Read the model definition and answer for the solid it produces. Units are mm, in the model's axes. A direction names the side the tool comes from. Round coordinates to 2 decimals unless told otherwise and drop trailing zeros. Order: outer loops, then holes, each group sorted by start corner. A loop starts at its lowest first (then second) coordinate and runs counter-clockwise, first axis right, second up. Notation, with made-up numbers: (84.5, 6) - (93.5, 6) arc R26 cw to (93.5, 26) - close; hole circle Ø5 at (-31, 52). An arc over 180 degrees is marked (long way). One line per question, with ' | ' between items. Start each with the question number.
1) The part is cut by section A-A, the plane y = -242.5. Give the vertices of the cut face in (x, z), plus the area to 3 significant figures.
2) Flat-ended cylindrical pins translate along their axes: pin 1 (5 mm diameter, centred on x = 10.5, z = 71.5, fed in from +Y); pin 2 (3 mm diameter, centred on x = -21, z = 16.5, fed in from +Y); pin 3 (21 mm diameter, centred on x = -3.5, z = 47, fed in from +Y); pin 4 (6 mm diameter, centred on x = 0, y = -400, fed in from +Z). Find the tip coordinate at first contact, or state that the pin passes through.
3) Straight lines are drawn through the part: line 1 (X direction, y = -400, z = 82.25); line 2 (Y direction, x = -5.5, z = 64); line 3 (Z direction, x = 3.5, y = -175). For each, find the intervals that lie inside material, in ascending order. Write a range as from..to.
4) The mould has two halves that part along Y. Classify faces 1 (the flat face through (0, -186, 15)), 2 (the cylindrical face through (0, -420, 82)), 3 (the flat face through (0, -192, 0)): pulls with the +Y half, pulls with the -Y half, needs draft (parallel to the pull), parting line crosses it, or undercut.
5) For faces 4 (the flat face through (0, -323, 75)), 5 (the flat face through (0, -192, 90)), 6 (the flat face through (0, -390, 75)), determine the directions among +Z, -Z, +X, -X, +Y, -Y from which every point of the face is accessible in a straight line to the end or side of a thin tool.
6) The part is cut by section D-D, the plane z = 5.5. Give the vertices of the cut face in (x, y), plus the area to 3 significant figures.
7) The part is cut by section B-B, the plane z = 26.5. Give the vertices of the cut face in (x, y).
8) The part is cut by section C-C, the plane x = 0. Count the separate pieces of the cut face and the enclosed holes in it, plus the area to 3 significant figures.
from build123d import *

# Parameters (mm, degrees)
SKETCH_1_R               = 5
EXTRUDE_1_DEPTH          = 90
CUT_EXTRUDE_1_DEPTH      = 431.581002832
CUT_EXTRUDE_1_DEPTH_BACK = 431.581002832
SKETCH_2_W               = 60
SKETCH_2_H               = 150
SKETCH_2_H_2             = 140.75
FILLET_1_R               = 3


with BuildPart() as part:
    # 草图1 → 凸台-拉伸1 (new body)
    with BuildSketch(Plane.XY):
        with BuildLine():
            Line((-29.990623535, -0.75), (-19.993749023, -400.5))
            ThreePointArc((-19.993749023, -400.5), (0, -420), (19.993749023, -400.5))
            Line((19.993749023, -400.5), (29.990623535, -0.75))
            ThreePointArc((29.990623535, -0.75), (0, 30), (-29.990623535, -0.75))
        make_face()
        with Locations(Location((0, 0, 0), (0, 0, 180))):
            Circle(SKETCH_1_R, mode=Mode.SUBTRACT)
        with Locations(Location((0, -400, 0), (0, 0, 180))):
            Circle(SKETCH_1_R, mode=Mode.SUBTRACT)
    extrude(amount=EXTRUDE_1_DEPTH)

    # 草图2 → 切除-拉伸1 (cut, two sides: drawn at the far end of the back side and taken through both)
    with BuildSketch(Plane(origin=(0, 0, 0), x_dir=(0, 0, -1), z_dir=(1, 0, 0)).offset(-CUT_EXTRUDE_1_DEPTH_BACK)):
        with Locations((-45, -445.75)):
            Rectangle(SKETCH_2_W, SKETCH_2_H)
        Polygon((-75, -20), (-15, -20), (-15, -80), align=None)
        Polygon((-75, -40), (-75, -100), (-15, -100), align=None)
        Polygon((-15, -330.75), (-75, -270.75), (-15, -270.75), align=None)
        Polygon((-15, -350.75), (-75, -290.75), (-75, -350.75), align=None)
        with Locations((-45, -185.375)):
            Rectangle(SKETCH_2_W, SKETCH_2_H_2)
    extrude(amount=CUT_EXTRUDE_1_DEPTH + CUT_EXTRUDE_1_DEPTH_BACK, mode=Mode.SUBTRACT)

    # 圆角1
    fillet_1_edges = [part.edges().sort_by_distance(p)[0] for p in [
        (0, -270.75, 75),
        (0, -270.75, 15),
        (0, -330.75, 15),
        (0, -255.75, 75),
        (0, -115, 75),
        (0, -115, 15),
        (0, -255.75, 15),
        (0, -350.75, 15),
        (0, -350.75, 75),
        (0, -290.75, 75),
        (0, -40, 75),
        (0, -100, 15),
        (0, -100, 75),
        (0, -80, 15),
        (0, -20, 75),
        (0, -20, 15),
    ]]
    fillet(fillet_1_edges, radius=FILLET_1_R)


solid = part.part
Values:
1) outline: (-23.94, 0) - (23.94, 0) - (23.94, 15) - (-23.94, 15) - close; (-23.94, 75) - (23.94, 75) - (23.94, 90) - (-23.94, 90) - close | area: 1,440 mm^2
2) pin 1: stops at y = 28.91 | pin 2: stops at y = 22.8 | pin 3: stops at y = 30 | pin 4: passes through
3) line 1: x = -20.01..-5, 5..20.01 | line 2: y = -370.75..-350.75, -301.75..-281.75, -270.75..-255.75, -115..-100, -51..-31, -20..29.49 | line 3: z = 0..15, 75..90
4) face 1: undercut | face 2: pulls with the -Y half | face 3: needs draft
5) face 4: +X, -X | face 5: +Z, +X, -X, +Y, -Y | face 6: +X, -X, -Y
6) outline: (-29.99, -0.75) - (-19.99, -400.5) arc R20 ccw to (19.99, -400.5) - (29.99, -0.75) arc R30 ccw (long way) to start; hole circle Ø10 at (0, -400); hole circle Ø10 at (0, 0) | area: 21,900 mm^2
7) outline: (-29.99, -0.75) - (-29.51, -20) - (29.51, -20) - (29.99, -0.75) arc R30 ccw (long way) to start; (-28.3, -68.5) - (-27.8, -88.5) - (27.8, -88.5) - (28.3, -68.5) - close; (-27.51, -100) - (-27.13, -115) - (27.13, -115) - (27.51, -100) - close; (-23.61, -255.75) - (-23.24, -270.75) - (23.24, -270.75) - (23.61, -255.75) - close; (-22.03, -319.25) - (-21.53, -339.25) - (21.53, -339.25) - (22.03, -319.25) - close; (-21.24, -350.75) - (-20.74, -370.75) - (20.74, -370.75) - (21.24, -350.75) - close; hole circle Ø10 at (0, 0)
8) separate pieces: 4 | enclosed holes: 5 | area: 20,800 mm^2
